Geometry check sheet. Reference: the model listing, model coordinates, mm. A direction names the side the tool comes from. Round coordinates to 2 decimals unless told otherwise and drop trailing zeros. Order: outer loops, then holes, each group sorted by start corner. A loop starts at its lowest first (then second) coordinate and runs counter-clockwise, first axis right, second up.
```python
from build123d import *

# Parameters (mm, degrees)
BOSS_EXTRUDE7_DEPTH     = 2
SKETCH8_R               = 3
BOSS_EXTRUDE8_DEPTH     = 2
SKETCH9_R               = 1.5
BOSS_EXTRUDE9_DEPTH     = 2
BOSS_EXTRUDE10_DEPTH    = 9
SKETCH12_W              = 14
SKETCH12_H              = 5
CUT_EXTRUDE5_DEPTH      = 10
CUT_EXTRUDE5_DEPTH_BACK = 10
SKETCH13_W              = 8.729840012
SKETCH13_H              = 32.4
CUT_EXTRUDE6_DEPTH      = 6.2


with BuildPart() as part:
    # Sketch7 → Boss-Extrude7 (new body)
    with BuildSketch(Plane(origin=(0, 0, 0), x_dir=(1, 0, 0), z_dir=(0, 1, 0))):
        with BuildLine():
            Line((30.48, 27.87), (-29.941284627, 27.87))
            ThreePointArc((-29.941284627, 27.87), (-33.058077828, 26.779680312), (-34.815550633, 23.984240056))
            ThreePointArc((-34.815550633, 23.984240056), (-37.522, 0), (-34.815550633, -23.984240056))
            ThreePointArc((-34.815550633, -23.984240056), (-33.058077828, -26.779680312), (-29.941284627, -27.87))
            Line((-29.941284627, -27.87), (30.48, -27.87))
            ThreePointArc((30.48, -27.87), (34.050723427, -26.374261545), (35.489363684, -22.780153375))
            ThreePointArc((35.489363684, -22.780153375), (34.068, 0), (35.489363684, 22.780153375))
            ThreePointArc((35.489363684, 22.780153375), (34.050723427, 26.374261545), (30.48, 27.87))
        make_face()
    extrude(amount=BOSS_EXTRUDE7_DEPTH)

    # Sketch8 → Boss-Extrude8 (add)
    with BuildSketch(Plane(origin=(0, 2, 0), x_dir=(1, 0, 0), z_dir=(0, 1, 0))):
        with Locations((-30.48, 20.32)):
            Circle(SKETCH8_R)
        with Locations((-30.48, -20.32)):
            Circle(SKETCH8_R)
        with Locations((30.48, -22.86)):
            Circle(SKETCH8_R)
        with Locations((30.48, 22.86)):
            Circle(SKETCH8_R)
    extrude(amount=BOSS_EXTRUDE8_DEPTH)

    # Sketch9 → Boss-Extrude9 (add)
    with BuildSketch(Plane(origin=(0, 4, 0), x_dir=(1, 0, 0), z_dir=(0, 1, 0))):
        with Locations((-30.48, 20.32)):
            Circle(SKETCH9_R)
        with Locations((30.48, 22.86)):
            Circle(SKETCH9_R)
        with Locations((30.48, -22.86)):
            Circle(SKETCH9_R)
        with Locations((-30.48, -20.32)):
            Circle(SKETCH9_R)
    extrude(amount=BOSS_EXTRUDE9_DEPTH)

    # Sketch10 → Boss-Extrude10 (add)
    with BuildSketch(Plane(origin=(0, 2, 0), x_dir=(1, 0, 0), z_dir=(0, 1, 0))):
        with BuildLine():
            Line((30.48, 27.87), (-29.941284627, 27.87))
            ThreePointArc((-29.941284627, 27.87), (-33.058077828, 26.779680312), (-34.815550633, 23.984240056))
            ThreePointArc((-34.815550633, 23.984240056), (-37.522, 0), (-34.815550633, -23.984240056))
            ThreePointArc((-34.815550633, -23.984240056), (-33.058077828, -26.779680312), (-29.941284627, -27.87))
            Line((-29.941284627, -27.87), (30.48, -27.87))
            ThreePointArc((30.48, -27.87), (34.050723427, -26.374261545), (35.489363684, -22.780153375))
            ThreePointArc((35.489363684, -22.780153375), (34.068, 0), (35.489363684, 22.780153375))
            ThreePointArc((35.489363684, 22.780153375), (34.050723427, 26.374261545), (30.48, 27.87))
        make_face()
        with BuildLine():
            Line((-29.941284627, -26.87), (30.48, -26.87))
            ThreePointArc((30.48, -26.87), (33.319950466, -25.691038917), (34.489980196, -22.847397183))
            ThreePointArc((34.489980196, -22.847397183), (33.068, 0), (34.489980196, 22.847397183))
            ThreePointArc((34.489980196, 22.847397183), (33.319950466, 25.691038917), (30.48, 26.87))
            Line((30.48, 26.87), (-29.941284627, 26.87))
            ThreePointArc((-29.941284627, 26.87), (-32.434719188, 25.997744249), (-33.840697431, 23.761392045))
            ThreePointArc((-33.840697431, 23.761392045), (-36.522, 0), (-33.840697431, -23.761392045))
            ThreePointArc((-33.840697431, -23.761392045), (-32.434719188, -25.997744249), (-29.941284627, -26.87))
        make_face(mode=Mode.SUBTRACT)
    extrude(amount=BOSS_EXTRUDE10_DEPTH)

    # Sketch12 → Cut-Extrude5 (cut, two sides)
    with BuildSketch(Plane(origin=(34.068, 0, 0), x_dir=(0, 0, -1), z_dir=(1, 0, 0))) as cut_extrude5_sk:
        with Locations((0, 7.1)):
            Rectangle(SKETCH12_W, SKETCH12_H)
    extrude(amount=CUT_EXTRUDE5_DEPTH, mode=Mode.SUBTRACT)
    extrude(cut_extrude5_sk.sketch, amount=-CUT_EXTRUDE5_DEPTH_BACK, mode=Mode.SUBTRACT)

    # Sketch13 → Cut-Extrude6 (cut)
    with BuildSketch(Plane(origin=(0, 11, 0), x_dir=(1, 0, 0), z_dir=(0, 1, 0))):
        with Locations((-37.029964161, 0)):
            Rectangle(SKETCH13_W, SKETCH13_H)
    extrude(amount=-CUT_EXTRUDE6_DEPTH, mode=Mode.SUBTRACT)


solid = part.part
```
(1) Sectioned sample at A-A, the plane y = 8.5. Record the cut outline in (x, z).
Returned:
outline: (-36.3, -16.2) arc R107.63 ccw to (-34.82, -23.98) arc R5 ccw to (-29.94, -27.87) - (30.48, -27.87) arc R5.01 ccw to (35.49, -22.78) arc R183.26 cw to (34.2, -7) - (33.2, -7) arc R184.26 ccw to (34.49, -22.85) arc R4.01 cw to (30.48, -26.87) - (-29.94, -26.87) arc R4 cw to (-33.84, -23.76) arc R106.63 cw to (-35.28, -16.2) - close; (-36.3, 16.2) - (-35.28, 16.2) arc R106.63 cw to (-33.84, 23.76) arc R4 cw to (-29.94, 26.87) - (30.48, 26.87) arc R4.01 cw to (34.49, 22.85) arc R184.26 ccw to (33.2, 7) - (34.2, 7) arc R183.26 cw to (35.49, 22.78) arc R5.01 ccw to (30.48, 27.87) - (-29.94, 27.87) arc R5 ccw to (-34.82, 23.98) arc R107.63 ccw to start
(2) Sectioned sample at B-B, the plane z = -3.5. Record the cut outline in (x, y), and give its area (3 significant figures).
Returned:
outline: (-37.47, 0) - (34.1, 0) - (34.1, 4.6) - (33.1, 4.6) - (33.1, 2) - (-36.46, 2) - (-36.46, 4.8) - (-37.47, 4.8) - close; (33.1, 9.6) - (34.1, 9.6) - (34.1, 11) - (33.1, 11) - close
area: 150 mm2
(3) Sectioned sample at D-D, the plane z = 10.5. Record the cut outline in (x, y).
Returned:
outline: (-37.01, 0) - (34.37, 0) - (34.37, 11) - (33.37, 11) - (33.37, 2) - (-36, 2) - (-36, 4.8) - (-37.01, 4.8) - close
(4) Set-up check for faces 5 (the cylindrical face through (-33.477, 2.986, -20.452)), 6 (the flat face through (1, 5, -27.87)): record each of +Z, -Z, +X, -X, +Y, -Y from which the full face is reachable in a straight line by a thin tool's end or side.
Returned:
face 5: +Y
face 6: -Z, +X, -X, +Y, -Y
(5) Material ranges on line 1 (Z direction, x = 7.5, y = 3.75); line 2 (X direction, y = 8, z = 26); line 3 (Y direction, x = -18, z = 2.5), recorded low to high.
Returned:
line 1: z = -27.87 to -26.87, 26.87 to 27.87
line 2: x = -33.84 to -32.43, 32.97 to 34.38
line 3: y = 0 to 2
(6) Sectioned sample at C-C, the plane x = 6. Record the cut outline in (y, z).
Returned:
outline: (0, -27.87) - (11, -27.87) - (11, -26.87) - (2, -26.87) - (2, 26.87) - (11, 26.87) - (11, 27.87) - (0, 27.87) - close
(7) Depth check by flat-ended pin: P1, Ø0.8, axis at x = 33.5, y = 7.5, coming from the +Z side; P2, Ø2, axis at x = 5.5, z = 10, coming from the -Y side; P3, Ø6, axis at y = 2.5, z = 14.5, coming from the -X side; P4, Ø3.5, axis at x = 31, z = -23.5, coming from the +Y side. Enter the tip coordinate at first touch or a pass-through.
Returned:
P1: stops at z = 27.13
P2: stops at y = 0
P3: stops at x = -36.91
P4: stops at y = 6
(8) Draft check along X on faces 1 (the cylindrical face through (28.099, 2.986, -21.035)), 2 (the cylindrical face through (-36.52, 4.44, -0.34)), 3 (the cylindrical face through (-33.02, 5.42, -26.81)), 4 (the flat face through (-37, 4.8, 0)). Enter one of: released by +X, released by -X, zero draft, split by the parting line, or undercut.
Returned:
face 1: undercut
face 2: undercut
face 3: released by -X
face 4: zero draft
